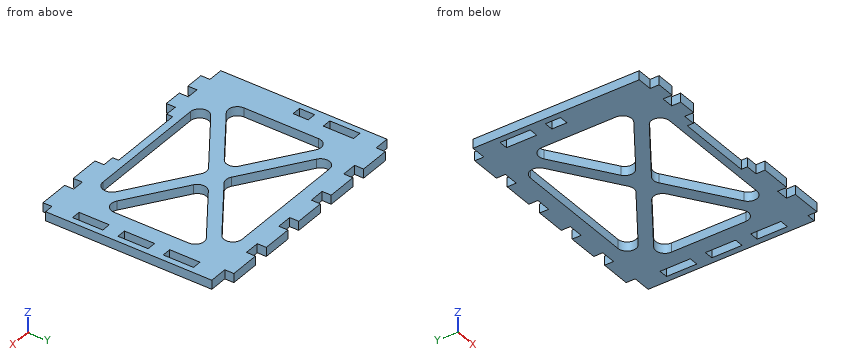
from build123d import *

# Parameters (mm, degrees)
SKETCH_1_W          = 3
SKETCH_1_H          = 10
SKETCH_1_H_2        = 5
EXTRUDE_1_DEPTH     = 3
CUT_EXTRUDE_1_DEPTH = 10
FILLET_1_R          = 3


with BuildPart() as part:
    # 草图1 → 凸台-拉伸1 (new body)
    with BuildSketch(Plane.XY):
        Polygon((-10.5, 27.5), (-10.5, 30.5), (-20.5, 30.5), (-20.5, 27.5), (-25.5, 27.5), (-25.5, 30.5), (-35.5, 30.5), (-35.5, 27.5), (-40.5, 27.5), (-40.5, -27.5), (-35.5, -27.5), (-35.5, -30.5), (-29.5, -30.5), (-29.5, -27.5), (-25.5, -27.5), (-25.5, -30.5), (-19.5, -30.5), (-19.5, -27.5), (-15.5, -27.5), (-15.5, -25.5), (9.5, -25.5), (9.5, -27.5), (13.5, -27.5), (13.5, -30.5), (23.5, -30.5), (23.5, -27.5), (27.5, -27.5), (27.5, -30.5), (37.5, -30.5), (37.5, -27.5), (40.5, -27.5), (40.5, 27.5), (34.5, 27.5), (34.5, 30.5), (24.5, 30.5), (24.5, 27.5), (19.5, 27.5), (19.5, 30.5), (9.5, 30.5), (9.5, 27.5), (4.5, 27.5), (4.5, 30.5), (-5.5, 30.5), (-5.5, 27.5), align=None)
        with Locations((37, 0)):
            Rectangle(SKETCH_1_W, SKETCH_1_H, mode=Mode.SUBTRACT)
        with Locations((37, 15)):
            Rectangle(SKETCH_1_W, SKETCH_1_H, mode=Mode.SUBTRACT)
        with Locations((37, -15)):
            Rectangle(SKETCH_1_W, SKETCH_1_H, mode=Mode.SUBTRACT)
        with Locations((-37, 2.5)):
            Rectangle(SKETCH_1_W, SKETCH_1_H_2, mode=Mode.SUBTRACT)
        with Locations((-37, 15)):
            Rectangle(SKETCH_1_W, SKETCH_1_H, mode=Mode.SUBTRACT)
    extrude(amount=EXTRUDE_1_DEPTH)

    # 草图2 → 切除-拉伸1 (cut)
    with BuildSketch(Plane.XY.offset(3)):
        Polygon((-30, 23), (30, 23), (0, 2.62962963), align=None)
        Polygon((-30, -23), (0, -2.62962963), (30, -23), align=None)
        Polygon((30, -18), (30, 18), (3.490909091, 0), align=None)
        Polygon((-30, -18), (-3.490909091, 0), (-30, 18), align=None)
    extrude(amount=-CUT_EXTRUDE_1_DEPTH, mode=Mode.SUBTRACT)

    # 圆角1
    fillet_1_edges = [part.edges().sort_by_distance(p)[0] for p in [
        (30, -18, 1.5),
        (3.490909091, 0, 1.5),
        (30, 18, 1.5),
        (30, -23, 1.5),
        (-30, -23, 1.5),
        (0, -2.62962963, 1.5),
        (-30, -18, 1.5),
        (-30, 18, 1.5),
        (-3.490909091, 0, 1.5),
        (30, 23, 1.5),
        (0, 2.62962963, 1.5),
        (-30, 23, 1.5),
    ]]
    fillet(fillet_1_edges, radius=FILLET_1_R)


solid = part.part
CAD build for the part. Positions are in the model's coordinates, mm. Round coordinates to 2 decimals unless told otherwise and drop trailing zeros. Write each loop counter-clockwise with the first axis right and the second up, starting at its lowest first coordinate (ties: lowest second). Pieces come first, ordered by that corner, then holes. Notation, with made-up numbers: M 17.25,-27.75 L 52.25,-27.75 A12 ccw 52.25,-13.75 Z; hole C 82,-33.75 d5. An arc over 180 degrees is marked long. Use a Markdown table: item, result. Add a question column.
1. Flat gauge pins, fed straight in: P1, Ø0.9, axis at y = -29.5, z = 1, coming from the -X side; P2, Ø1.5, axis at x = 22, z = 2, coming from the +Y side; P3, Ø0.9, axis at y = -28.5, z = 1.5, coming from the +X side. Where does each tip first touch, or does it go through?
2. Drill centre lines: probe 1 along X at (y, z) = (-28, 2.4); probe 2 along X at (y, z) = (9, 0.35); probe 3 along X at (y, z) = (14, 1.15). Where is each one in solid material? Low to high.
3. Slice it at A-A on y = 1.5. Give the cut face in (x, z), then the cut area to 3 significant figures.
4. Slice it at C-C on z = 0.95. Give the number of separate pieces and of enclosed holes in the cut face, then the cut area to 3 significant figures.
5. Slice it at B-B on x = -9. Give the cut face in (y, z), then the cut area to 3 significant figures.
Reply:
| question | item | result |
|---|---|---|
| 1 | P1 | stops at x = -35.5 |
| 1 | P2 | stops at y = 27.5 |
| 1 | P3 | stops at x = 37.5 |
| 2 | probe 1 | x = -35.5 to -29.5, -25.5 to -19.5, 13.5 to 23.5, 27.5 to 37.5 |
| 2 | probe 2 | x = -40.5 to -30, -16.75 to -9.38, 9.38 to 16.75, 30 to 40.5 |
| 2 | probe 3 | x = -40.5 to -38.5, -35.5 to -29.5, -24.11 to -16.75, 16.75 to 24.11, 29.5 to 35.5, 38.5 to 40.5 |
| 3 | outline | M -40.5,0 L -38.5,0 L -38.5,3 L -40.5,3 Z; M -35.5,0 L -30,0 L -30,3 L -35.5,3 Z; M -6.23,0 L 6.23,0 L 6.23,3 L -6.23,3 Z; M 30,0 L 35.5,0 L 35.5,3 L 30,3 Z; M 38.5,0 L 40.5,0 L 40.5,3 L 38.5,3 Z |
| 3 | area | 82.4 mm^2 |
| 4 | separate pieces | 1 |
| 4 | enclosed holes | 9 |
| 4 | area | 2,450 mm^2 |
| 5 | outline | M -25.5,0 L -23,0 L -23,3 L -25.5,3 Z; M -8.74,0 L -3.74,0 L -3.74,3 L -8.74,3 Z; M 3.74,0 L 8.74,0 L 8.74,3 L 3.74,3 Z; M 23,0 L 27.5,0 L 27.5,3 L 23,3 Z |
| 5 | area | 51.0 mm^2 |
